```python
from build123d import *

# Parameters (mm, degrees)
F1_DEPTH = 6.35
F3_DEPTH = 6.351
F4_R     = 2.54


with BuildPart() as f1:
    # F0 (on Top) → F1 (new body)
    with BuildSketch(Plane.XY):
        Polygon((-38.1, 203.2), (-57.15, 0), (57.15, 0), (38.1, 203.2), align=None)
    extrude(amount=F1_DEPTH)

    # F2 (on face) → F3 (cut, through all)
    with BuildSketch(Plane.XY.offset(6.35)):
        Polygon((0, 50.8), (-50.8, 0), (50.8, 0), align=None)
    extrude(amount=-F3_DEPTH, mode=Mode.SUBTRACT)

    # F4
    f4_edges = [f1.edges().sort_by_distance(p)[0] for p in [
        (-38.1, 203.2, 3.175),
        (38.1, 203.2, 3.175),
        (0, 50.8, 3.175),
        (-50.8, 0, 3.175),
        (-57.15, 0, 3.175),
        (50.8, 0, 3.175),
        (57.15, 0, 3.175),
    ]]
    fillet(f4_edges, radius=F4_R)


solid = f1.part
```
Could you check a few things on this model? Use its own coordinates, in mm. A direction names the side the tool comes from. Coordinates: 2 decimals unless noted, no trailing zeros. Loops run counter-clockwise (first coordinate to the right, second up) from the corner with the lowest first, then second, coordinate; pieces in that order, holes last.
1) Thinking about a two-plate mould opening in X: for faces 3 (the face through (-1, 103, 6.35)), 4 (the face through (-0.028, 49.748, 3.131)), 5 (the face through (-47.473, 103.224, 3.131)), which applies, released by +X, released by -X, zero draft, split by the parting line, or undercut?
Reported:
face 3: zero draft
face 4: undercut
face 5: released by -X
2) Imagine slicing it at A-A (z = 3). List the corners of the cut face in (x, y) for me.
Reported:
outline: (-56.89, 2.78) arc R2.54 ccw to (-54.36, 0) - (-51.85, 0) arc R2.54 ccw to (-50.06, 0.74) - (-1.8, 49) arc R2.54 cw to (1.8, 49) - (50.06, 0.74) arc R2.54 ccw to (51.85, 0) - (54.36, 0) arc R2.54 ccw to (56.89, 2.78) - (38.32, 200.9) arc R2.54 ccw to (35.79, 203.2) - (-35.79, 203.2) arc R2.54 ccw to (-38.32, 200.9) - close
3) Which directions (+Z, -Z, +X, -X, +Y, -Y) give clear straight access to the entire face, cutting with the end or side of a thin tool? Please do faces 1 (the face through (-25.6, 25.2, 3.2)), 2 (the face through (1, 203.2, 3)).
Reported:
face 1: +Z, -Z, -Y
face 2: +Z, -Z, +X, -X, +Y
4) Please list where these lines run through material, in increasing order: line 1 along X through (y, z) = (41, 4); line 2 along X through (y, z) = (106, 6.25); line 3 along Y through (x, z) = (4.5, 0.75).
Reported:
line 1: x = -53.31 to -9.8, 9.8 to 53.31
line 2: x = -47.21 to 47.21
line 3: y = 46.3 to 203.2
5) Imagine slicing it at B-B (y = 13). List the corners of the cut face in (x, z) for me, and give its area (3 significant figures).
Reported:
outline: (-55.93, 0) - (-37.8, 0) - (-37.8, 6.35) - (-55.93, 6.35) - close; (37.8, 0) - (55.93, 0) - (55.93, 6.35) - (37.8, 6.35) - close
area: 230 mm2
6) Will these pins go through, and if not, where does the flat tip stop? pin 1 Ø1 at (x, z) = (24.5, 5.5) entering from -Y; pin 2 Ø2 at (y, z) = (72.5, 4) entering from +X; pin 3 Ø1.5 at (y, z) = (102.5, 2) entering from +X.
Reported:
pin 1: stops at y = 25.8
pin 2: stops at x = 50.45
pin 3: stops at x = 47.61
7) Imagine slicing it at C-C (x = -12). List the corners of the cut face in (y, z) for me, and give its area (3 significant figures).
Reported:
outline: (38.8, 0) - (203.2, 0) - (203.2, 6.35) - (38.8, 6.35) - close
area: 1,040 mm2
8) Imagine slicing it at D-D (y = 176). List the corners of the cut face in (x, z) for me.
Reported:
outline: (-40.65, 0) - (40.65, 0) - (40.65, 6.35) - (-40.65, 6.35) - close
